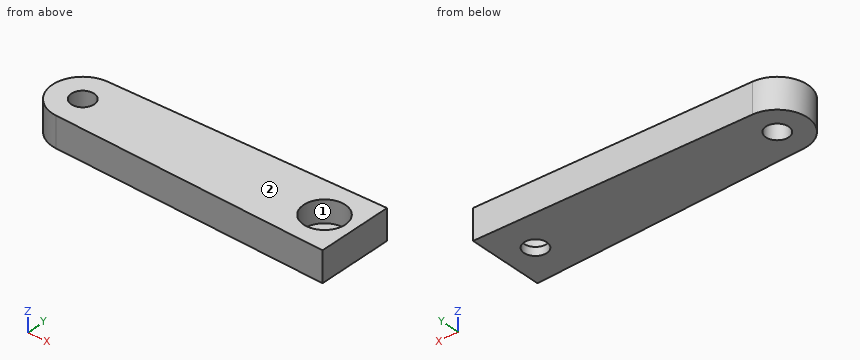
```python
from build123d import *

# Parameters (mm, degrees)
SKETCH_1_R          = 1.5
EXTRUDE_1_DEPTH     = 4
SKETCH_2_R          = 2.75
CUT_EXTRUDE_1_DEPTH = 2.9


with BuildPart() as part:
    # 草图1 → 凸台-拉伸1 (new body)
    with BuildSketch(Plane.XY):
        with BuildLine():
            Line((-32.110897558, 3.998462421), (4, 5))
            Line((4, 5), (4, -5))
            Line((4, -5), (-32.110897558, -3.998462421))
            ThreePointArc((-32.110897558, -3.998462421), (-36, 0), (-32.110897558, 3.998462421))
        make_face()
        Circle(SKETCH_1_R, mode=Mode.SUBTRACT)
        with Locations((-32, 0)):
            Circle(SKETCH_1_R, mode=Mode.SUBTRACT)
    extrude(amount=EXTRUDE_1_DEPTH)

    # 草图2 → 切除-拉伸1 (cut)
    with BuildSketch(Plane.XY.offset(4)):
        Circle(SKETCH_2_R)
    extrude(amount=-CUT_EXTRUDE_1_DEPTH, mode=Mode.SUBTRACT)


solid = part.part
```
For this review, take the finished solid that the model builds, in its own axes (mm). Face numbers are marked on the shaded views. A direction names the side the tool comes from. Give positions to 0.01 mm unless a question says otherwise; leave off trailing zeros. Write each loop counter-clockwise with the first axis right and the second up, starting at its lowest first coordinate (ties: lowest second). Pieces come first, ordered by that corner, then holes. Notation, with made-up numbers: M -15,15 L 16,15 A29 cw 16,49 Z; hole C 71.5,-8.5 d6. An arc over 180 degrees is marked long. One line per item, written item: value.
1) Take a section at D-D, the plane y = -2.25. Write out the cut boundary in (x, z), then the cut area to 3 significant figures.
Results are:
outline: M -35.31,0 L 4,0 L 4,4 L 1.58,4 L 1.58,1.1 L -1.58,1.1 L -1.58,4 L -35.31,4 Z
area: 148 mm²
2) For P1, Ø2, axis at x = -4, z = 3, coming from the -Y side; P2, Ø1, axis at x = -12.5, z = 2.5, coming from the +Y side; P3, Ø2, axis at x = 0, z = 2.5, coming from the +Y side, all flat-tipped, find the tip position at first contact; note any pin that passes through.
Results are:
P1: stops at y = -4.81
P2: stops at y = 4.56
P3: stops at y = 4.92
3) For line 1 (X direction, y = -0.5, z = 3); line 2 (X direction, y = -1.25, z = 3.35); line 3 (Z direction, x = -2, y = 0.5), list the stretches that pass through material, from the lowest coordinate up. Write a range as from..to.
Results are:
line 1: x = -35.97..-33.41, -30.59..-2.7, 2.7..4
line 2: x = -35.8..-32.83, -31.17..-2.45, 2.45..4
line 3: z = 0..1.1
4) For the marked faces 1 and 2, list the 3-axis set-ups (+Z, -Z, +X, -X, +Y, -Y) from which the entire face can be reached by the end or side of a thin tool; tool diameter is ignored.
Results are:
face 1: +Z
face 2: +Z, +X, -X, +Y, -Y
5) Take a section at B-B, the plane z = 3.4. Write out the cut boundary in (x, y), then the cut area to 3 significant figures.
Results are:
outline: M -32.11,-4 L 4,-5 L 4,5 L -32.11,4 A4 ccw Z; hole C -32,0 d3; hole C 0,0 d5.5
area: 318 mm²
6) Take a section at A-A, the plane y = 0. Write out the cut boundary in (x, z).
Results are:
outline: M -36,0 L -33.5,0 L -33.5,4 L -36,4 Z; M -30.5,0 L -1.5,0 L -1.5,1.1 L -2.75,1.1 L -2.75,4 L -30.5,4 Z; M 1.5,0 L 4,0 L 4,4 L 2.75,4 L 2.75,1.1 L 1.5,1.1 Z
7) Take a section at C-C, the plane x = 0. Write out the cut boundary in (y, z), then the cut area to 3 significant figures.
Results are:
outline: M -4.89,0 L -1.5,0 L -1.5,1.1 L -2.75,1.1 L -2.75,4 L -4.89,4 Z; M 1.5,0 L 4.89,0 L 4.89,4 L 2.75,4 L 2.75,1.1 L 1.5,1.1 Z
area: 19.9 mm²
